```python
from build123d import *

# Parameters (mm, degrees)
SKETCH3_W           = 183.5200292
SKETCH3_H           = 183.5200292
BOSS_EXTRUDE1_DEPTH = 3.0988
SKETCH4_R           = 1.524
CUT_EXTRUDE1_DEPTH  = 260.555013045
CUT_EXTRUDE2_REACH  = 261.555
SKETCH5_R           = 6.35
SKETCH5_W           = 69.85
SKETCH5_H           = 95.25
SKETCH7_R           = 1.6002
CUT_EXTRUDE6_DEPTH  = 2.54


with BuildPart() as part:
    # Sketch3 → Boss-Extrude1 (new body)
    with BuildSketch(Plane(origin=(0, 0, 0), x_dir=(1, 0, 0), z_dir=(0, 1, 0))):
        with Locations((91.7600146, 91.7600146)):
            Rectangle(SKETCH3_W, SKETCH3_H)
    extrude(amount=BOSS_EXTRUDE1_DEPTH)

    # Sketch4 → Cut-Extrude1 (cut, through all)
    with BuildSketch(Plane(origin=(0, 3.0988, 0), x_dir=(1, 0, 0), z_dir=(0, 1, 0))):
        with Locations(Location((5.200015, 102.6820146, 0), (0, 0, 270))):
            Circle(SKETCH4_R)
        with Locations(Location((11.550015, 102.6820146, 0), (0, 0, 270))):
            Circle(SKETCH4_R)
        with Locations(Location((11.550015, 80.8380146, 0), (0, 0, 90))):
            Circle(SKETCH4_R)
        with Locations(Location((5.200015, 80.8380146, 0), (0, 0, 90))):
            Circle(SKETCH4_R)
        with Locations(Location((178.3200142, 80.8380146, 0), (0, 0, 270))):
            Circle(SKETCH4_R)
        with Locations(Location((171.9700142, 80.8380146, 0), (0, 0, 270))):
            Circle(SKETCH4_R)
        with Locations(Location((171.9700142, 102.6820146, 0), (0, 0, 90))):
            Circle(SKETCH4_R)
        with Locations(Location((178.3200142, 102.6820146, 0), (0, 0, 90))):
            Circle(SKETCH4_R)
        with Locations(Location((80.8380146, 178.3130292, 0), (0, 0, 270))):
            Circle(SKETCH4_R)
        with Locations(Location((80.8380146, 171.9630292, 0), (0, 0, 270))):
            Circle(SKETCH4_R)
        with Locations(Location((102.6820146, 171.9630292, 0), (0, 0, 90))):
            Circle(SKETCH4_R)
        with Locations(Location((102.6820146, 178.3130292, 0), (0, 0, 90))):
            Circle(SKETCH4_R)
        with Locations(Location((102.6820146, 5.207, 0), (0, 0, 270))):
            Circle(SKETCH4_R)
        with Locations(Location((102.6820146, 11.557, 0), (0, 0, 270))):
            Circle(SKETCH4_R)
        with Locations(Location((80.8380146, 11.557, 0), (0, 0, 90))):
            Circle(SKETCH4_R)
        with Locations(Location((80.8380146, 5.207, 0), (0, 0, 90))):
            Circle(SKETCH4_R)
        with BuildLine():
            Line((17.646015, 101.1580146), (30.346015, 101.1580146))
            ThreePointArc((30.346015, 101.1580146), (31.870015, 102.6820146), (30.346015, 104.2060146))
            Line((30.346015, 104.2060146), (17.646015, 104.2060146))
            ThreePointArc((17.646015, 104.2060146), (16.122015, 102.6820146), (17.646015, 101.1580146))
        make_face()
        with BuildLine():
            Line((17.646015, 79.3140146), (30.346015, 79.3140146))
            ThreePointArc((30.346015, 79.3140146), (31.870015, 80.8380146), (30.346015, 82.3620146))
            Line((30.346015, 82.3620146), (17.646015, 82.3620146))
            ThreePointArc((17.646015, 82.3620146), (16.122015, 80.8380146), (17.646015, 79.3140146))
        make_face()
        with BuildLine():
            Line((165.8740142, 82.3620146), (153.1740142, 82.3620146))
            ThreePointArc((153.1740142, 82.3620146), (151.6500142, 80.8380146), (153.1740142, 79.3140146))
            Line((153.1740142, 79.3140146), (165.8740142, 79.3140146))
            ThreePointArc((165.8740142, 79.3140146), (167.3980142, 80.8380146), (165.8740142, 82.3620146))
        make_face()
        with BuildLine():
            Line((165.8740142, 104.2060146), (153.1740142, 104.2060146))
            ThreePointArc((153.1740142, 104.2060146), (151.6500142, 102.6820146), (153.1740142, 101.1580146))
            Line((153.1740142, 101.1580146), (165.8740142, 101.1580146))
            ThreePointArc((165.8740142, 101.1580146), (167.3980142, 102.6820146), (165.8740142, 104.2060146))
        make_face()
        with BuildLine():
            Line((79.3140146, 153.1670292), (79.3140146, 165.8670292))
            ThreePointArc((79.3140146, 165.8670292), (80.8380146, 167.3910292), (82.3620146, 165.8670292))
            Line((82.3620146, 165.8670292), (82.3620146, 153.1670292))
            ThreePointArc((82.3620146, 153.1670292), (80.8380146, 151.6430292), (79.3140146, 153.1670292))
        make_face()
        with BuildLine():
            Line((101.1580146, 153.1670292), (101.1580146, 165.8670292))
            ThreePointArc((101.1580146, 165.8670292), (102.6820146, 167.3910292), (104.2060146, 165.8670292))
            Line((104.2060146, 165.8670292), (104.2060146, 153.1670292))
            ThreePointArc((104.2060146, 153.1670292), (102.6820146, 151.6430292), (101.1580146, 153.1670292))
        make_face()
        with BuildLine():
            Line((104.2060146, 30.353), (104.2060146, 17.653))
            ThreePointArc((104.2060146, 17.653), (102.6820146, 16.129), (101.1580146, 17.653))
            Line((101.1580146, 17.653), (101.1580146, 30.353))
            ThreePointArc((101.1580146, 30.353), (102.6820146, 31.877), (104.2060146, 30.353))
        make_face()
        with BuildLine():
            Line((82.3620146, 30.353), (82.3620146, 17.653))
            ThreePointArc((82.3620146, 17.653), (80.8380146, 16.129), (79.3140146, 17.653))
            Line((79.3140146, 17.653), (79.3140146, 30.353))
            ThreePointArc((79.3140146, 30.353), (80.8380146, 31.877), (82.3620146, 30.353))
        make_face()
    extrude(amount=-CUT_EXTRUDE1_DEPTH, mode=Mode.SUBTRACT)

    # Sketch5 → Cut-Extrude2 (cut, up to next)
    with BuildSketch(Plane(origin=(0, 3.0988, 0), x_dir=(1, 0, 0), z_dir=(0, 1, 0)), mode=Mode.PRIVATE) as cut_extrude2_sk1:
        with Locations(Location((170.8200292, 151.7700292, 0), (0, 0, 90))):
            Circle(SKETCH5_R)
    cut_extrude2_tool1 = extrude(cut_extrude2_sk1.sketch, amount=-CUT_EXTRUDE2_REACH, mode=Mode.PRIVATE) & part.part
    # Sketch5 → Cut-Extrude2 (cut, up to next)
    with BuildSketch(Plane(origin=(0, 3.0988, 0), x_dir=(1, 0, 0), z_dir=(0, 1, 0)), mode=Mode.PRIVATE) as cut_extrude2_sk2:
        with Locations(Location((170.8200292, 170.8200292, 0), (0, 0, 90))):
            Circle(SKETCH5_R)
    cut_extrude2_tool2 = extrude(cut_extrude2_sk2.sketch, amount=-CUT_EXTRUDE2_REACH, mode=Mode.PRIVATE) & part.part
    # Sketch5 → Cut-Extrude2 (cut, up to next)
    with BuildSketch(Plane(origin=(0, 3.0988, 0), x_dir=(1, 0, 0), z_dir=(0, 1, 0)), mode=Mode.PRIVATE) as cut_extrude2_sk3:
        with Locations(Location((151.7700292, 170.8200292, 0), (0, 0, 90))):
            Circle(SKETCH5_R)
    cut_extrude2_tool3 = extrude(cut_extrude2_sk3.sketch, amount=-CUT_EXTRUDE2_REACH, mode=Mode.PRIVATE) & part.part
    # Sketch5 → Cut-Extrude2 (cut, up to next)
    with BuildSketch(Plane(origin=(0, 3.0988, 0), x_dir=(1, 0, 0), z_dir=(0, 1, 0)), mode=Mode.PRIVATE) as cut_extrude2_sk4:
        with Locations(Location((170.8200292, 31.75, 0), (0, 0, 270))):
            Circle(SKETCH5_R)
    cut_extrude2_tool4 = extrude(cut_extrude2_sk4.sketch, amount=-CUT_EXTRUDE2_REACH, mode=Mode.PRIVATE) & part.part
    # Sketch5 → Cut-Extrude2 (cut, up to next)
    with BuildSketch(Plane(origin=(0, 3.0988, 0), x_dir=(1, 0, 0), z_dir=(0, 1, 0)), mode=Mode.PRIVATE) as cut_extrude2_sk5:
        with Locations(Location((12.7, 31.75, 0), (0, 0, 90))):
            Circle(SKETCH5_R)
    cut_extrude2_tool5 = extrude(cut_extrude2_sk5.sketch, amount=-CUT_EXTRUDE2_REACH, mode=Mode.PRIVATE) & part.part
    # Sketch5 → Cut-Extrude2 (cut, up to next)
    with BuildSketch(Plane(origin=(0, 3.0988, 0), x_dir=(1, 0, 0), z_dir=(0, 1, 0)), mode=Mode.PRIVATE) as cut_extrude2_sk6:
        with Locations(Location((12.7, 12.7, 0), (0, 0, 90))):
            Circle(SKETCH5_R)
    cut_extrude2_tool6 = extrude(cut_extrude2_sk6.sketch, amount=-CUT_EXTRUDE2_REACH, mode=Mode.PRIVATE) & part.part
    # Sketch5 → Cut-Extrude2 (cut, up to next)
    with BuildSketch(Plane(origin=(0, 3.0988, 0), x_dir=(1, 0, 0), z_dir=(0, 1, 0)), mode=Mode.PRIVATE) as cut_extrude2_sk7:
        with Locations(Location((31.75, 12.7, 0), (0, 0, 90))):
            Circle(SKETCH5_R)
    cut_extrude2_tool7 = extrude(cut_extrude2_sk7.sketch, amount=-CUT_EXTRUDE2_REACH, mode=Mode.PRIVATE) & part.part
    # Sketch5 → Cut-Extrude2 (cut, up to next)
    with BuildSketch(Plane(origin=(0, 3.0988, 0), x_dir=(1, 0, 0), z_dir=(0, 1, 0)), mode=Mode.PRIVATE) as cut_extrude2_sk8:
        with Locations(Location((151.7700292, 12.7, 0), (0, 0, 270))):
            Circle(SKETCH5_R)
    cut_extrude2_tool8 = extrude(cut_extrude2_sk8.sketch, amount=-CUT_EXTRUDE2_REACH, mode=Mode.PRIVATE) & part.part
    # Sketch5 → Cut-Extrude2 (cut, up to next)
    with BuildSketch(Plane(origin=(0, 3.0988, 0), x_dir=(1, 0, 0), z_dir=(0, 1, 0)), mode=Mode.PRIVATE) as cut_extrude2_sk9:
        with Locations(Location((31.75, 170.8200292, 0), (0, 0, 270))):
            Circle(SKETCH5_R)
    cut_extrude2_tool9 = extrude(cut_extrude2_sk9.sketch, amount=-CUT_EXTRUDE2_REACH, mode=Mode.PRIVATE) & part.part
    # Sketch5 → Cut-Extrude2 (cut, up to next)
    with BuildSketch(Plane(origin=(0, 3.0988, 0), x_dir=(1, 0, 0), z_dir=(0, 1, 0)), mode=Mode.PRIVATE) as cut_extrude2_sk10:
        with Locations(Location((12.7, 170.8200292, 0), (0, 0, 270))):
            Circle(SKETCH5_R)
    cut_extrude2_tool10 = extrude(cut_extrude2_sk10.sketch, amount=-CUT_EXTRUDE2_REACH, mode=Mode.PRIVATE) & part.part
    # Sketch5 → Cut-Extrude2 (cut, up to next)
    with BuildSketch(Plane(origin=(0, 3.0988, 0), x_dir=(1, 0, 0), z_dir=(0, 1, 0)), mode=Mode.PRIVATE) as cut_extrude2_sk11:
        with Locations(Location((12.7, 151.7700292, 0), (0, 0, 270))):
            Circle(SKETCH5_R)
    cut_extrude2_tool11 = extrude(cut_extrude2_sk11.sketch, amount=-CUT_EXTRUDE2_REACH, mode=Mode.PRIVATE) & part.part
    # Sketch5 → Cut-Extrude2 (cut, up to next)
    with BuildSketch(Plane(origin=(0, 3.0988, 0), x_dir=(1, 0, 0), z_dir=(0, 1, 0)), mode=Mode.PRIVATE) as cut_extrude2_sk12:
        with Locations(Location((170.8200292, 12.7, 0), (0, 0, 270))):
            Circle(SKETCH5_R)
    cut_extrude2_tool12 = extrude(cut_extrude2_sk12.sketch, amount=-CUT_EXTRUDE2_REACH, mode=Mode.PRIVATE) & part.part
    # Sketch5 → Cut-Extrude2 (cut, up to next)
    with BuildSketch(Plane(origin=(0, 3.0988, 0), x_dir=(1, 0, 0), z_dir=(0, 1, 0)), mode=Mode.PRIVATE) as cut_extrude2_sk13:
        with Locations((91.7600146, 91.7600146)):
            Rectangle(SKETCH5_W, SKETCH5_H)
    cut_extrude2_tool13 = extrude(cut_extrude2_sk13.sketch, amount=-CUT_EXTRUDE2_REACH, mode=Mode.PRIVATE) & part.part
    add(cut_extrude2_tool1.solids().sort_by_distance((170.820029, 3.0988, -151.770029))[0], mode=Mode.SUBTRACT)
    add(cut_extrude2_tool2.solids().sort_by_distance((170.820029, 3.0988, -170.820029))[0], mode=Mode.SUBTRACT)
    add(cut_extrude2_tool3.solids().sort_by_distance((151.770029, 3.0988, -170.820029))[0], mode=Mode.SUBTRACT)
    add(cut_extrude2_tool4.solids().sort_by_distance((170.820029, 3.0988, -31.75))[0], mode=Mode.SUBTRACT)
    add(cut_extrude2_tool5.solids().sort_by_distance((12.7, 3.0988, -31.75))[0], mode=Mode.SUBTRACT)
    add(cut_extrude2_tool6.solids().sort_by_distance((12.7, 3.0988, -12.7))[0], mode=Mode.SUBTRACT)
    add(cut_extrude2_tool7.solids().sort_by_distance((31.75, 3.0988, -12.7))[0], mode=Mode.SUBTRACT)
    add(cut_extrude2_tool8.solids().sort_by_distance((151.770029, 3.0988, -12.7))[0], mode=Mode.SUBTRACT)
    add(cut_extrude2_tool9.solids().sort_by_distance((31.75, 3.0988, -170.820029))[0], mode=Mode.SUBTRACT)
    add(cut_extrude2_tool10.solids().sort_by_distance((12.7, 3.0988, -170.820029))[0], mode=Mode.SUBTRACT)
    add(cut_extrude2_tool11.solids().sort_by_distance((12.7, 3.0988, -151.770029))[0], mode=Mode.SUBTRACT)
    add(cut_extrude2_tool12.solids().sort_by_distance((170.820029, 3.0988, -12.7))[0], mode=Mode.SUBTRACT)
    add(cut_extrude2_tool13.solids().sort_by_distance((91.760015, 3.0988, -91.760015))[0], mode=Mode.SUBTRACT)

    # Sketch7 → Cut-Extrude6 (cut)
    with BuildSketch(Plane(origin=(0, 3.0988, 0), x_dir=(1, 0, 0), z_dir=(0, 1, 0))):
        with Locations(Location((7.4828146, 43.3120292, 0), (0, 0, 270))):
            Circle(SKETCH7_R)
        with Locations(Location((176.0372146, 43.3120292, 0), (0, 0, 270))):
            Circle(SKETCH7_R)
    extrude(amount=-CUT_EXTRUDE6_DEPTH, mode=Mode.SUBTRACT)


solid = part.part
```
Here's how the part is built. I have some questions about the finished solid (model axes, mm). Round coordinates to 2 decimals unless told otherwise and drop trailing zeros. Loops run counter-clockwise (first coordinate to the right, second up) from the corner with the lowest first, then second, coordinate; pieces in that order, holes last.
1. Thinking about a two-plate mould opening in Z: for faces 1 (the face through (157.97, 1.57, -169.44)), 2 (the face through (50, 3.099, -93)), which applies, released by +Z, released by -Z, zero draft, split by the parting line, or undercut?
Answers:
face 1: undercut
face 2: zero draft
2. Will these pins go through, and if not, where does the flat tip stop? pin 1 (5 mm diameter, centred on x = 178.32, z = -80.84, fed in from +Y); pin 2 (1 mm diameter, centred on x = 26, z = -80, fed in from -Y).
Answers:
pin 1: stops at y = 3.1
pin 2: passes through
3. Suppose I cut it at B-B, the plane z = -108. Please give me the cut outline in (x, y), and give its area (3 significant figures).
Answers:
outline: (0, 0) - (56.84, 0) - (56.84, 3.1) - (0, 3.1) - close; (126.69, 0) - (183.52, 0) - (183.52, 3.1) - (126.69, 3.1) - close
area: 352 mm2
4. If I drill on probe 1 along Z at (x, y) = (125, 2.1); probe 2 along X at (y, z) = (2.95, -45); probe 3 along Z at (x, y) = (150, 0.3), over which ranges is the centre line in solid material (lowest first)?
Answers:
probe 1: z = -183.52 to -139.39, -44.14 to 0
probe 2: x = 0 to 56.84, 126.69 to 183.52
probe 3: z = -183.52 to -176.92, -164.72 to -18.8, -6.6 to 0
5. Suppose I cut it at C-C, the plane y = 2.5. Give the number of separate pieces and of enclosed holes in the cut face, and give its area (3 significant figures).
Answers:
separate pieces: 1
enclosed holes: 39
area: 25,000 mm2
6. Suppose I cut it at A-A, the plane x = 119. Please give me the cut outline in (y, z).
Answers:
outline: (0, -183.52) - (3.1, -183.52) - (3.1, -139.39) - (0, -139.39) - close; (0, -44.14) - (3.1, -44.14) - (3.1, 0) - (0, 0) - close
